Check sheet for the drawn part. Datum: minimum x, y, z corner. Units: mm. Round coordinates to 2 decimals unless told otherwise and drop trailing zeros. Write each loop counter-clockwise with the first axis right and the second up, starting at its lowest first coordinate (ties: lowest second). Pieces come first, ordered by that corner, then holes. Notation, with made-up numbers: M -32.75,83 L 7.25,83 A34 ccw 7.25,117 Z; hole C 27.5,27.5 d2. An arc over 180 degrees is marked long. One line per item, written item: value. Start each with the question number.
Item 1: Section check A-A, the plane z = 12.5. Record the cut outline in (x, y).
Item 2: Section check B-B, the plane x = 12.5. Record the cut outline in (y, z), then the cut area to 3 significant figures.
Item 3: Gauge pin test, flat ends, axial feed: pin 1 (1.5 mm diameter, centred on x = 10.5, y = 2, fed in from -Z); pin 2 (2 mm diameter, centred on x = 19, z = 10, fed in from -Y). Record the tip position at first contact, or that the pin passes through.
Item 4: Draft check along Z on the marked faces 1, 2 and 3. Enter one of: +Z half, -Z half, draft (parallel to the pull), parting line (faces both ways), or undercut.
Item 5: Thickness scan on probe 1 along X at (y, z) = (1, 12.5); probe 2 along X at (y, z) = (2.95, 20.75); probe 3 along Z at (x, y) = (8.75, 0.8) (1 decimal). Record the ranges inside material, lowest first. Write a range as from..to.
Item 6: Section check D-D, the plane z = 8.25. Record the cut outline in (x, y) (1 decimal).
Item 7: Section check C-C, the plane y = 2.7. Record the cut outline in (x, z).
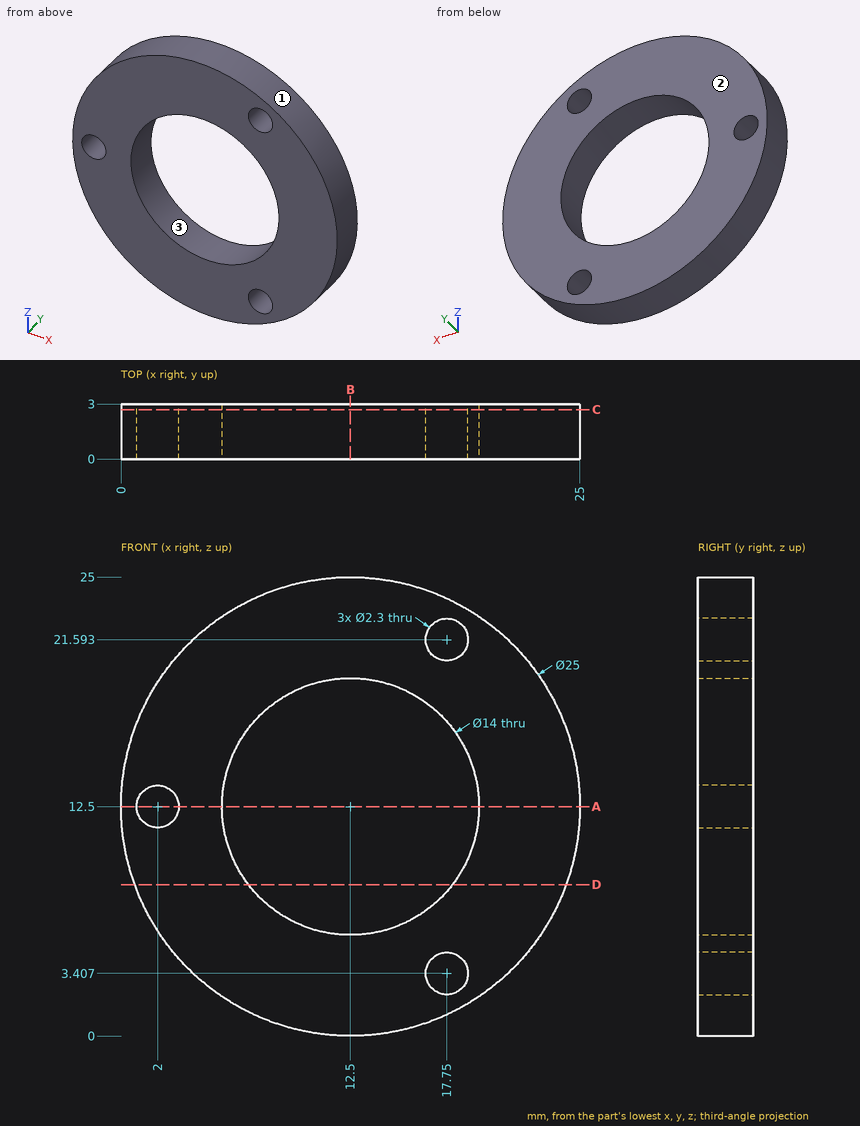
Response values:
1. outline: M 0,0 L 0.85,0 L 0.85,3 L 0,3 Z; M 3.15,0 L 5.5,0 L 5.5,3 L 3.15,3 Z; M 19.5,0 L 25,0 L 25,3 L 19.5,3 Z
2. outline: M 0,0 L 3,0 L 3,5.5 L 0,5.5 Z; M 0,19.5 L 3,19.5 L 3,25 L 0,25 Z
2. area: 33.0 mm2
3. pin 1: stops at z = 0.06
3. pin 2: stops at y = 0
4. face 1: parting line
4. face 2: draft
4. face 3: undercut
5. probe 1: x = 0..0.85, 3.15..5.5, 19.5..25
5. probe 2: x = 3.11..16.97, 18.53..21.89
5. probe 3: z = 0.6..6.6, 18.4..24.4
6. outline: M 0.7,0 L 6.9,0 L 6.9,3 L 0.7,3 Z; M 18.1,0 L 24.3,0 L 24.3,3 L 18.1,3 Z
7. outline: C 12.5,12.5 d25; hole C 2,12.5 d2.3; hole C 12.5,12.5 d14; hole C 17.75,3.41 d2.3; hole C 17.75,21.59 d2.3
